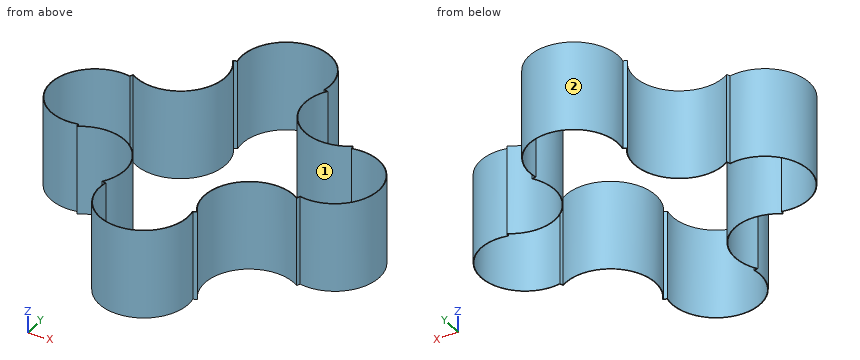
from build123d import *

# Parameters (mm, degrees)
F1_DEPTH = 300
F2_T     = -2.5


with BuildPart() as f1:
    # F0 (on Top) → F1 (new body)
    with BuildSketch(Plane.XY):
        with BuildLine():
            ThreePointArc((-158.7704400152, 367.1402284923), (-176.7766952966, 176.7766952966), (-367.1402284923, 158.7704400152))
            ThreePointArc((-367.1402284923, 158.7704400152), (-369.5518130045, 153.073372946), (-371.875, 147.3396904266))
            ThreePointArc((-371.875, 147.3396904266), (-550, 0), (-371.875, -147.3396904266))
            ThreePointArc((-371.875, -147.3396904266), (-369.5518130045, -153.073372946), (-367.1402284923, -158.7704400152))
            ThreePointArc((-367.1402284923, -158.7704400152), (-176.7766952966, -176.7766952966), (-158.7704400152, -367.1402284923))
            ThreePointArc((-158.7704400152, -367.1402284923), (-153.073372946, -369.5518130045), (-147.3396904266, -371.875))
            ThreePointArc((-147.3396904266, -371.875), (0, -550), (147.3396904266, -371.875))
            ThreePointArc((147.3396904266, -371.875), (153.073372946, -369.5518130045), (158.7704400152, -367.1402284923))
            ThreePointArc((158.7704400152, -367.1402284923), (176.7766952966, -176.7766952966), (367.1402284923, -158.7704400152))
            ThreePointArc((367.1402284923, -158.7704400152), (369.5518130045, -153.073372946), (371.875, -147.3396904266))
            ThreePointArc((371.875, -147.3396904266), (550, 0), (371.875, 147.3396904266))
            ThreePointArc((371.875, 147.3396904266), (369.5518130045, 153.073372946), (367.1402284923, 158.7704400152))
            ThreePointArc((367.1402284923, 158.7704400152), (176.7766952966, 176.7766952966), (158.7704400152, 367.1402284923))
            ThreePointArc((158.7704400152, 367.1402284923), (153.073372946, 369.5518130045), (147.3396904266, 371.875))
            ThreePointArc((147.3396904266, 371.875), (0, 550), (-147.3396904266, 371.875))
            ThreePointArc((-147.3396904266, 371.875), (-153.073372946, 369.5518130045), (-158.7704400152, 367.1402284923))
        make_face()
    extrude(amount=F1_DEPTH)

    # F2
    f2_openings = [f1.faces().sort_by_distance(p)[0] for p in [
        (0, 0, 300),
        (0, 0, 0),
    ]]
    offset(amount=F2_T, openings=f2_openings, kind=Kind.INTERSECTION)


solid = f1.part
For this review, take the finished solid that the model builds, in its own axes (mm). Face numbers are marked on the shaded views. Give positions to 0.01 mm unless a question says otherwise; leave off trailing zeros. Loops run counter-clockwise (first coordinate to the right, second up) from the corner with the lowest first, then second, coordinate; pieces in that order, holes last.
Item 1: For line 1 along Y through (x, z) = (-400, 124.5); line 2 along Y through (x, z) = (151.5, 183), list the stretches that pass through material, from the lowest coordinate up.
Item 2: Insertion check: pin 1 (3 mm diameter, centred on x = -10.5, z = 215, fed in from -Y); pin 2 (8 mm diameter, centred on x = -80.5, z = 79.5, fed in from +Y); pin 3 (3 mm diameter, centred on y = -216.5, z = 123.5, fed in from -X). Each pin has a flat end and moves straight along its axis. Give the tip position at first contact, or say it passes through.
Item 3: Take a section at A-A, the plane y = -400. State the section outline as (x, z) points, and give its area (3 significant figures).
Item 4: Draft analysis for pull direction X (two halves, no side actions). For the marked faces 1 and 2, state which applies: +X half, -X half, draft (parallel to the pull), parting line (faces both ways), or undercut.
Calculated:
1. line 1: y = -150 to -147.5, 147.5 to 150
1. line 2: y = -370.2 to -367.5, -360.34 to -355.29, -210.39 to -205.35, 205.35 to 210.39, 355.29 to 360.34, 367.5 to 370.2
2. pin 1: stops at y = -549.73
2. pin 2: stops at y = 529.03
2. pin 3: stops at x = -149.06
3. outline: (-150, 0) - (-147.5, 0) - (-147.5, 300) - (-150, 300) - close; (147.5, 0) - (150, 0) - (150, 300) - (147.5, 300) - close
3. area: 1,500 mm2
4. face 1: undercut
4. face 2: parting line
